For this review, use the dimensioned drawing (mm, ordinates from the lowest corner) and the shaded views. Round coordinates to 2 decimals unless told otherwise and drop trailing zeros. Loops run counter-clockwise (first coordinate to the right, second up) from the corner with the lowest first, then second, coordinate; pieces in that order, holes last. Notation, with made-up numbers: M 56,88 L 77,88 A20 cw 77,108 Z; hole C 88,-18.75 d10. An arc over 180 degrees is marked long. Answer as a JSON object with one key per item and string values. Group by question number.
Item 1: Consider section C-C (y = 2.25). Give the boundary of the cut face in (x, z).
Item 2: To check wall thickness, follow line 1 (Y direction, x = 32.5, z = 0.9); line 2 (Z direction, x = 67.5, y = 3.6). State the ranges of each line that lie inside material, in increasing order.
Item 3: Consider section A-A (z = 0.55). Give the boundary of the cut face in (x, y).
Item 4: Consider section B-B (x = 21). Give the boundary of the cut face in (y, z).
Item 5: Insertion check: P1, Ø2.5, axis at x = 47, y = 3, coming from the -Z side. The pin has a flat end and moves straight along its axis. Give the tip position at first contact, or say it passes through.
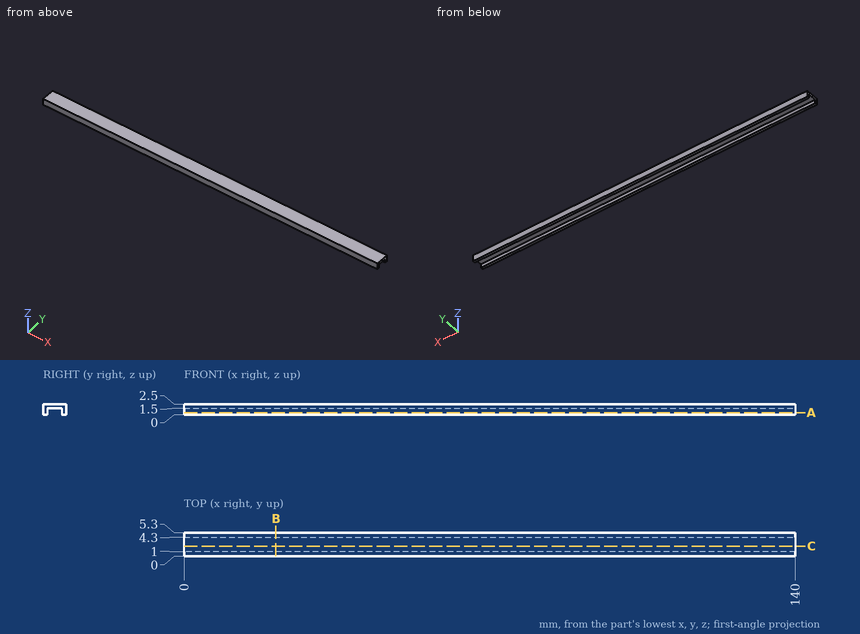
Geometry results:
{
 "1": {"outline": "M 0,1.5 L 140,1.5 L 140,2.5 L 0,2.5 Z"},
 "2": {"line 1": "y = 0 to 1, 4.3 to 5.3", "line 2": "z = 1.5 to 2.5"},
 "3": {"outline": "M 0,0 L 140,0 L 140,1 L 0,1 Z; M 0,4.3 L 140,4.3 L 140,5.3 L 0,5.3 Z"},
 "4": {"outline": "M 0,0 L 1,0 L 1,1.5 L 4.3,1.5 L 4.3,0 L 5.3,0 L 5.3,2.5 L 0,2.5 Z"},
 "5": {"P1": "stops at z = 1.5"}
}
